from build123d import *

# Parameters (mm, degrees)
F0_R     = 14
F0_R_2   = 9.45
F1_DEPTH = 6
F3_DEPTH = 6


# Not quite as in the source:
# - a feature names something its author has since deleted; it is built from what else it names


with BuildPart() as f1:
    # F0 (on Top) → F1 (new body)
    with BuildSketch(Plane.XY):
        Circle(F0_R)
        Circle(F0_R_2, mode=Mode.SUBTRACT)
    extrude(amount=F1_DEPTH)

    # F2 (on Top) → F3 (join)
    with BuildSketch(Plane.XY):
        with BuildLine():
            ThreePointArc((7.1208542294, 12.0537726478), (5.7261776623, 13.9509775601), (6.1307398604, 16.2706410345))
            Line((6.1307398604, 16.2706410345), (12.124355653, 25.5))
            ThreePointArc((12.124355653, 25.5), (10.4510884103, 34.4532067527), (1.3471506281, 34.1738301594))
            ThreePointArc((1.3471506281, 34.1738301594), (0, 33.6520673478), (-1.3471506281, 34.1738301594))
            ThreePointArc((-1.3471506281, 34.1738301594), (-10.4510884103, 34.4532067527), (-12.124355653, 25.5))
            Line((-12.124355653, 25.5), (-6.1307398604, 16.2706410345))
            ThreePointArc((-6.1307398604, 16.2706410345), (-5.7261776623, 13.9509775601), (-7.1208542294, 12.0537726478))
            ThreePointArc((-7.1208542294, 12.0537726478), (0, 14), (7.1208542294, 12.0537726478))
        make_face()
        Polygon((-6.2786841774, 27.625), (0, 31.25), (6.2786841774, 27.625), (6.2786841774, 20.375), (0, 16.75), (-6.2786841774, 20.375), align=None, mode=Mode.SUBTRACT)
        with BuildLine():
            ThreePointArc((17.1561584019, -2.8259440541), (14.9449898058, -2.016473458), (13.9993004391, 0.1399543354))
            ThreePointArc((13.9993004391, 0.1399543354), (13.9998251087, 0.0699780419), (14, 0))
            ThreePointArc((14, 0), (12.0892151717, -7.0605153163), (6.8784462097, -12.1937269832))
            ThreePointArc((6.8784462097, -12.1937269832), (9.2188121436, -11.9345041022), (11.0254185415, -13.4446969803))
            Line((11.0254185415, -13.4446969803), (16.02146997, -23.25))
            ThreePointArc((16.02146997, -23.25), (24.6118080845, -26.2775114368), (28.9218297486, -18.2535817464))
            ThreePointArc((28.9218297486, -18.2535817464), (29.1435452131, -16.8260336739), (30.2689803767, -15.920248413))
            ThreePointArc((30.2689803767, -15.920248413), (35.0628964948, -8.1756953159), (28.145825623, -2.25))
            Line((28.145825623, -2.25), (17.1561584019, -2.8259440541))
        make_face()
        Polygon((27.0632938683, -15.625), (20.7846096908, -19.25), (14.5059255134, -15.625), (14.5059255134, -8.375), (20.7846096908, -4.75), (27.0632938683, -8.375), align=None, mode=Mode.SUBTRACT)
        with BuildLine():
            ThreePointArc((-6.8784462097, -12.1937269832), (-12.124355653, -7), (-13.9993004391, 0.1399543354))
            ThreePointArc((-13.9993004391, 0.1399543354), (-14.9449898058, -2.016473458), (-17.1561584019, -2.8259440541))
            Line((-17.1561584019, -2.8259440541), (-28.145825623, -2.25))
            ThreePointArc((-28.145825623, -2.25), (-35.0628964948, -8.1756953159), (-30.2689803767, -15.920248413))
            ThreePointArc((-30.2689803767, -15.920248413), (-29.1435452131, -16.8260336739), (-28.9218297486, -18.2535817464))
            ThreePointArc((-28.9218297486, -18.2535817464), (-24.6118080845, -26.2775114368), (-16.02146997, -23.25))
            Line((-16.02146997, -23.25), (-11.0254185415, -13.4446969803))
            ThreePointArc((-11.0254185415, -13.4446969803), (-9.2188121436, -11.9345041022), (-6.8784462097, -12.1937269832))
        make_face()
        Polygon((-27.0632938683, -15.625), (-27.0632938683, -8.375), (-20.7846096908, -4.75), (-14.5059255134, -8.375), (-14.5059255134, -15.625), (-20.7846096908, -19.25), align=None, mode=Mode.SUBTRACT)
    extrude(amount=F3_DEPTH)


solid = f1.part
Model file for the job. Use its own axes, mm. A direction names the side the tool comes from. Give positions to 0.01 mm unless a question says otherwise; leave off trailing zeros. Order: outer loops, then holes, each group sorted by start corner. A loop starts at its lowest first (then second) coordinate and runs counter-clockwise, first axis right, second up. Notation, with made-up numbers: M 54.25,42 L 63.25,42 A33 ccw 63.25,76 Z; hole C -9,-1.75 d7. An arc over 180 degrees is marked long. Put each result on its own line as item: value. Start each with the question number.
(1) Tool access for faces 1 (the face through (13.5, -18.3, 3)), 2 (the face through (3.1, 29.46, 2.96)), 3 (the face through (2.4, 9.4, 0)), 4 (the face through (14.97, -2.04, 2.96)): list every direction of +Z, -Z, +X, -X, +Y, -Y with a clear straight run to the whole face (end or side of a thin tool).
(2) Band-saw the part on C-C on z = 1.6. Count the separate pieces of the cut face and the enclosed holes in it, then the cut area to 3 significant figures.
(3) Band-saw the part on B-B on y = -20.5. Give the cut face in (x, z), then the cut area to 3 significant figures.
(4) Band-saw the part on A-A on x = 22.5. Give the cut face in (y, z).
(5) Pull direction X, two halves, no side cores. Call faces 5 (the face through (-23.97, -6.59, 2.96)), 6 (the face through (12.174, 6.913, 2.958)), 7 (the face through (-9.251, -11.944, 2.958)), 8 (the face through (-9.17, 20.95, 2.96)): released by +X, released by -X, zero draft, split by the parting line, or undercut.
(6) Drill centre lines: L1, parallel to Y at x = 0, z = 2.5; L2, parallel to Y at x = -4, z = 1.5; L3, parallel to Y at x = -20, z = 1.4. Where is each one in solid material? Low to high. Write a range as [from, to].
(7) Pin check, flat tips, straight feed: pin 1 Ø1.8 at (y, z) = (-11, 4) entering from +X; pin 2 Ø3 at (y, z) = (-11, 4) entering from -X; pin 3 Ø1 at (y, z) = (8.5, 3.5) entering from +X; pin 4 Ø15 at (x, y) = (0, 0) entering from +Z (3 decimals). Stop position of each tip, or through.
Results below:
1. face 1: +Z, -Z, -Y
1. face 2: +Z, -Z
1. face 3: -Z, +X, -X, +Y, -Y
1. face 4: +Z, -Z, +Y
2. separate pieces: 1
2. enclosed holes: 4
2. area: 1,250 mm2
3. outline: M -29.04,0 L -14.62,0 L -14.62,6 L -29.04,6 Z; M 14.62,0 L 29.04,0 L 29.04,6 L 14.62,6 Z
3. area: 173 mm2
4. outline: M -26.74,0 L -18.26,0 L -18.26,6 L -26.74,6 Z; M -5.74,0 L -2.55,0 L -2.55,6 L -5.74,6 Z
5. face 5: undercut
5. face 6: released by +X
5. face 7: undercut
5. face 8: released by -X
6. L1: y = [-14, -9.45], [9.45, 16.75], [31.25, 33.65]
6. L2: y = [-13.42, -8.56], [8.56, 19.06], [28.94, 35.69]
6. L3: y = [-26.43, -18.8], [-5.2, -2.68]
7. pin 1: stops at x = 35.09
7. pin 2: stops at x = -35.14
7. pin 3: stops at x = 11.49
7. pin 4: passes through
